Read the model definition and answer for the solid it produces. Units are mm, in the model's axes. Coordinates: 2 decimals unless noted, no trailing zeros. Loops run counter-clockwise (first coordinate to the right, second up) from the corner with the lowest first, then second, coordinate; pieces in that order, holes last. Notation, with made-up numbers: M 48,-39 L 62,-39 A21 cw 62,-19 Z; hole C -4,-4.5 d4. An arc over 180 degrees is marked long. Use one line per item in the form item = value. Start each with the question number.
1. The part is cut by section A-A (x = 4078.75). Give the vertices of the cut face in (y, z).
2. The part is cut by section C-C (x = 4073.75). Give the vertices of the cut face in (y, z), plus the area to 3 significant figures.
3. For a pull along X with two mould halves and no side action, classify faces 1 (the flat face through (4079.712, -3186, 8)), 2 (the flat face through (4071, -3186, 6)), 3 (the cylindrical face through (4074.503, -3176.949, 7.972)) as released by +X, released by -X, zero draft, split by the parting line, or undercut.
4. The part is cut by section B-B (z = 8.6). Give the vertices of the cut face in (x, y).
5. Find the intervals of material crossed by probe 1 along X at (y, z) = (-3177, 8.75); probe 2 along Y at (x, z) = (4073.25, 8.1), in increasing order. Write a range as [from, to].
from build123d import *

# Parameters (mm, degrees)
EXTRUDE_START   = 6
SKETCH_4_W      = 17.619983613
SKETCH_4_H      = 20.199783613
SKETCH_4_R      = 1
EXTRUDE_1_DEPTH = 4


with BuildPart() as part:
    # 草图4 → 凸台-拉伸1 (new body)
    with BuildSketch(Plane.XY.offset(EXTRUDE_START)):
        with Locations((4070.90198202, -3186.21042393)):
            Rectangle(SKETCH_4_W, SKETCH_4_H)
        with Locations((4073.549032956, -3177.249070092)):
            Circle(SKETCH_4_R, mode=Mode.SUBTRACT)
        with Locations((4078.449868123, -3177.249070092)):
            Circle(SKETCH_4_R, mode=Mode.SUBTRACT)
    extrude(amount=EXTRUDE_1_DEPTH)


solid = part.part
Computed values:
q1.outline = M -3196.31,6 L -3178.2,6 L -3178.2,10 L -3196.31,10 Z; M -3176.3,6 L -3176.11,6 L -3176.11,10 L -3176.3,10 Z
q2.outline = M -3196.31,6 L -3178.23,6 L -3178.23,10 L -3196.31,10 Z; M -3176.27,6 L -3176.11,6 L -3176.11,10 L -3176.27,10 Z
q2.area = 73.0 mm²
q3.face_1 = released by +X
q3.face_2 = zero draft
q3.face_3 = undercut
q4.outline = M 4062.09,-3196.31 L 4079.71,-3196.31 L 4079.71,-3176.11 L 4062.09,-3176.11 Z; hole C 4073.55,-3177.25 d2; hole C 4078.45,-3177.25 d2
q5.probe_1 = [4062.09, 4072.58], [4074.52, 4077.48], [4079.42, 4079.71]
q5.probe_2 = [-3196.31, -3178.2], [-3176.29, -3176.11]
